Source: CAD feature listing. Evaluate the final solid. Frame: model axes, mm. A direction names the side the tool comes from. Coordinates: 2 decimals unless noted, no trailing zeros. Write each loop counter-clockwise with the first axis right and the second up, starting at its lowest first coordinate (ties: lowest second). Pieces come first, ordered by that corner, then holes. Notation, with made-up numbers: (59, -32) -> (81, -32) arc R27 ccw to (81, -16) -> close; hole circle Ø4 at (43.5, 50). An arc over 180 degrees is marked (long way). One line per item, written item: value. Start each with the question number.
1. Section query B-B, the plane z = 10.25. Output: boundary loops of the cut face in (x, y).
2. Section query D-D, the plane z = 17.5. Output: boundary loops of the cut face in (x, y).
3. Access query for faces 5 (the cylindrical face through (93.505, 9.492, 25.353)), 6 (the cylindrical face through (8, 32, 15)), 7 (the flat face through (49, 58, 30)), 8 (the flat face through (54, 57, 15)). Directions: +Z, -Z, +X, -X, +Y, -Y. A direction counts if a zero-diameter tool reaches every point of the face in a straight line with its end or side. Return the directions, or none.
4. Section query C-C, the plane x = 99. Output: boundary loops of the cut face in (y, z) (3 decimals).
5. First-contact query: P1, Ø5.5, axis at x = 99, y = 57.75, coming from the +Z side; P2, Ø9, axis at x = 45, z = 13.5, coming from the -Y side; P3, Ø3.5, axis at x = 8.5, y = 55.5, coming from the +Z side. Flat tips, straight axial feed; report the tip coordinate or a pass-through.
6. Mould query, pull axis X, two halves, no side actions, for faces 1 (the cylindrical face through (6.57, 61.02, 10.44)), 2 (the flat face through (106, 34, 15)), 3 (the flat face through (95, 9, 20.6)), 4 (the flat face through (52, 67, 15)). Classes: released by +X, released by -X, zero draft, split by the parting line, or undercut.
7. Line query: line 1 (Y direction, x = 7, z = 26.25); line 2 (X direction, y = 23.5, z = 12.5); line 3 (Y direction, x = 9, z = 16). Output: solid intervals per line, ascending.
8. Section query A-A, the plane y = 9.25. Output: boundary loops of the cut face in (x, z) (3 decimals), and give its area (3 significant figures).
from build123d import *

# Parameters (mm, degrees)
P_IDAT_VYSUNUT_M1_DEPTH = 30


# Read off the part's stored shape, not the designer's step: Válcové zahloubení pro M6 šrouby s vnitřním šestihranem1
with BuildPart() as part:
    # Skica1 → Přidat vysunutím1 (new body)
    with BuildSketch(Plane.XY):
        Polygon((0, 0), (0, 67), (106, 67), (106, 0), (92, 0), (92, 57), (14, 57), (14, 0), align=None)
    extrude(amount=P_IDAT_VYSUNUT_M1_DEPTH)

    # Skica2 → Odebrat rotací1 (revolve, cut)
    with BuildSketch(Plane(origin=(0, 0, 0), x_dir=(-1, 0, 0), z_dir=(0, 0, -1))):
        Polygon((-114, 32), (-114, 19), (-104, 19), (-104, 17), (-2, 17), (-2, 19), (8, 19), (8, 32), align=None)
    revolve(axis=Axis((113.408800735, 32, 0), (-1, 0, 0)), mode=Mode.SUBTRACT)

    # V_lcov_ zahlouben_ pro M6 _rouby s v 2 → Válcové zahloubení pro M6 šrouby s vnitřním šestihranem1 (revolve, cut)
    with BuildSketch(Plane(origin=(99, 9.25, 0), x_dir=(1, 0, 0), z_dir=(0, -1, 0))):
        Polygon((0, 0), (3.3, 0), (3.3, 20.6), (5.5, 20.6), (5.5, 29.975), (5.525, 30), (0, 30), align=None)
    revolve(axis=Axis((99, 9.25, 0), (0, 0, 1)), mode=Mode.SUBTRACT)

    # V_lcov_ zahlouben_ pro M6 _rouby s v 3 o → V_lcov_ zahlouben_ pro M6 _rouby s v 3 (revolve, cut)
    with BuildSketch(Plane(origin=(7, 57.75, 0), x_dir=(1, 0, 0), z_dir=(0, -1, 0))):
        Polygon((0, 30), (0, 0), (3.3, 0), (3.3, 20.6), (5.5, 20.6), (5.5, 29.975), (5.525, 30), align=None)
    revolve(axis=Axis((7, 57.75, 0), (0, 0, 1)), mode=Mode.SUBTRACT)

    # V_lcov_ zahlouben_ pro M6 _rouby s v 4 o → V_lcov_ zahlouben_ pro M6 _rouby s v 4 (revolve, cut)
    with BuildSketch(Plane(origin=(99, 57.75, 0), x_dir=(1, 0, 0), z_dir=(0, -1, 0))):
        Polygon((0, 30), (0, 0), (3.3, 0), (3.3, 20.6), (5.5, 20.6), (5.5, 29.975), (5.525, 30), align=None)
    revolve(axis=Axis((99, 57.75, 0), (0, 0, 1)), mode=Mode.SUBTRACT)

    # V_lcov_ zahlouben_ pro M6 _rouby s v 5 o → V_lcov_ zahlouben_ pro M6 _rouby s v 5 (revolve, cut)
    with BuildSketch(Plane(origin=(7, 9.25, 0), x_dir=(1, 0, 0), z_dir=(0, -1, 0))):
        Polygon((0, 30), (0, 0), (3.3, 0), (3.3, 20.6), (5.5, 20.6), (5.5, 29.975), (5.525, 30), align=None)
    revolve(axis=Axis((7, 9.25, 0), (0, 0, 1)), mode=Mode.SUBTRACT)


solid = part.part
Computed values:
1. outline: (0, 0) -> (14, 0) -> (14, 21.05) -> (2, 21.05) -> (2, 24) -> (0, 24) -> close; (0, 40) -> (2, 40) -> (2, 42.95) -> (14, 42.95) -> (14, 57) -> (92, 57) -> (92, 42.95) -> (104, 42.95) -> (104, 40) -> (106, 40) -> (106, 67) -> (0, 67) -> close; (92, 0) -> (106, 0) -> (106, 24) -> (104, 24) -> (104, 21.05) -> (92, 21.05) -> close; hole circle Ø6.6 at (7, 9.25); hole circle Ø6.6 at (7, 57.75); hole circle Ø6.6 at (99, 9.25); hole circle Ø6.6 at (99, 57.75)
2. outline: (0, 0) -> (14, 0) -> (14, 57) -> (92, 57) -> (92, 0) -> (106, 0) -> (106, 67) -> (0, 67) -> close; hole circle Ø6.6 at (7, 9.25); hole circle Ø6.6 at (7, 57.75); hole circle Ø6.6 at (99, 9.25); hole circle Ø6.6 at (99, 57.75)
3. face 5: +Z
3. face 6: -Z
3. face 7: +Z, +X, -X, +Y, -Y
3. face 8: +Z, -Z, -Y
4. outline: (0, 0) -> (5.95, 0) -> (5.95, 20.6) -> (3.75, 20.6) -> (3.75, 29.975) -> (3.725, 30) -> (0, 30) -> close; (12.55, 0) -> (17, 0) arc R15 cw to (47, 0) -> (54.45, 0) -> (54.45, 20.6) -> (52.25, 20.6) -> (52.25, 29.975) -> (52.225, 30) -> (14.775, 30) -> (14.75, 29.975) -> (14.75, 20.6) -> (12.55, 20.6) -> close; (61.05, 0) -> (67, 0) -> (67, 30) -> (63.275, 30) -> (63.25, 29.975) -> (63.25, 20.6) -> (61.05, 20.6) -> close
5. P1: passes through
5. P2: stops at y = 57
5. P3: stops at z = 20.6
6. face 1: undercut
6. face 2: released by +X
6. face 3: undercut
6. face 4: zero draft
7. line 1: y = 0 to 3.75, 14.75 to 52.25, 63.25 to 67
7. line 2: x = 0 to 14, 92 to 106
7. line 3: y = 0 to 6.63, 11.87 to 55.13, 60.37 to 67
8. outline: (0, 0) -> (3.7, 0) -> (3.7, 20.6) -> (1.5, 20.6) -> (1.5, 29.975) -> (1.475, 30) -> (0, 30) -> close; (10.3, 0) -> (14, 0) -> (14, 30) -> (12.525, 30) -> (12.5, 29.975) -> (12.5, 20.6) -> (10.3, 20.6) -> close; (92, 0) -> (95.7, 0) -> (95.7, 20.6) -> (93.5, 20.6) -> (93.5, 29.975) -> (93.475, 30) -> (92, 30) -> close; (102.3, 0) -> (106, 0) -> (106, 30) -> (104.525, 30) -> (104.5, 29.975) -> (104.5, 20.6) -> (102.3, 20.6) -> close
8. area: 361 mm²
